Verification items for this drawing (mm, ordinates from the low corner). A direction names the side the tool comes from. Round coordinates to 2 decimals unless told otherwise and drop trailing zeros. Write each loop counter-clockwise with the first axis right and the second up, starting at its lowest first coordinate (ties: lowest second). Pieces come first, ordered by that corner, then holes.
Item 1: Cross-section at A-A (z = 27.5). Enter the section's corners in (x, y).
Item 2: Depth check by flat-ended pin: P1, Ø15, axis at x = 23.5, y = 23.5, coming from the -Z side; P2, Ø3.5, axis at x = 4.5, y = 26, coming from the +Z side; P3, Ø8, axis at y = 35.5, z = 17, coming from the -X side; P4, Ø4, axis at x = 44.5, z = 23, coming from the +Y side. Enter the tip coordinate at first touch or a pass-through.
Item 3: Cross-section at B-B (z = 37.5). State how many separate pieces and enclosed holes the cut face has, then the cut area to 3 significant figures.
Item 4: Cross-section at D-D (y = 10.5). Enter the section's corners in (x, z).
Item 5: Scan lines: probe 1 along Z at (x, y) = (20.5, 49.5); probe 2 along X at (y, z) = (26.5, 56.5); probe 3 along X at (y, z) = (47, 38) (1 decimal). Record each from-to range of solid material in increasing order.
Item 6: Draft check along Z on the marked faces 1, 2, 3 and 4. Enter one of: pulls with the +Z half, pulls with the -Z half, needs draft (parallel to the pull), parting line crosses it, or undercut.
Item 7: Access from +Z, -Z, +X, -X, +Y, -Y to the whole of each face (thin tool, end or side, straight path). Record for the marked faces 5 and 6.
Item 8: Cross-section at C-C (x = 35.5). Enter the section's corners in (y, z), then the cut area to 3 significant figures.
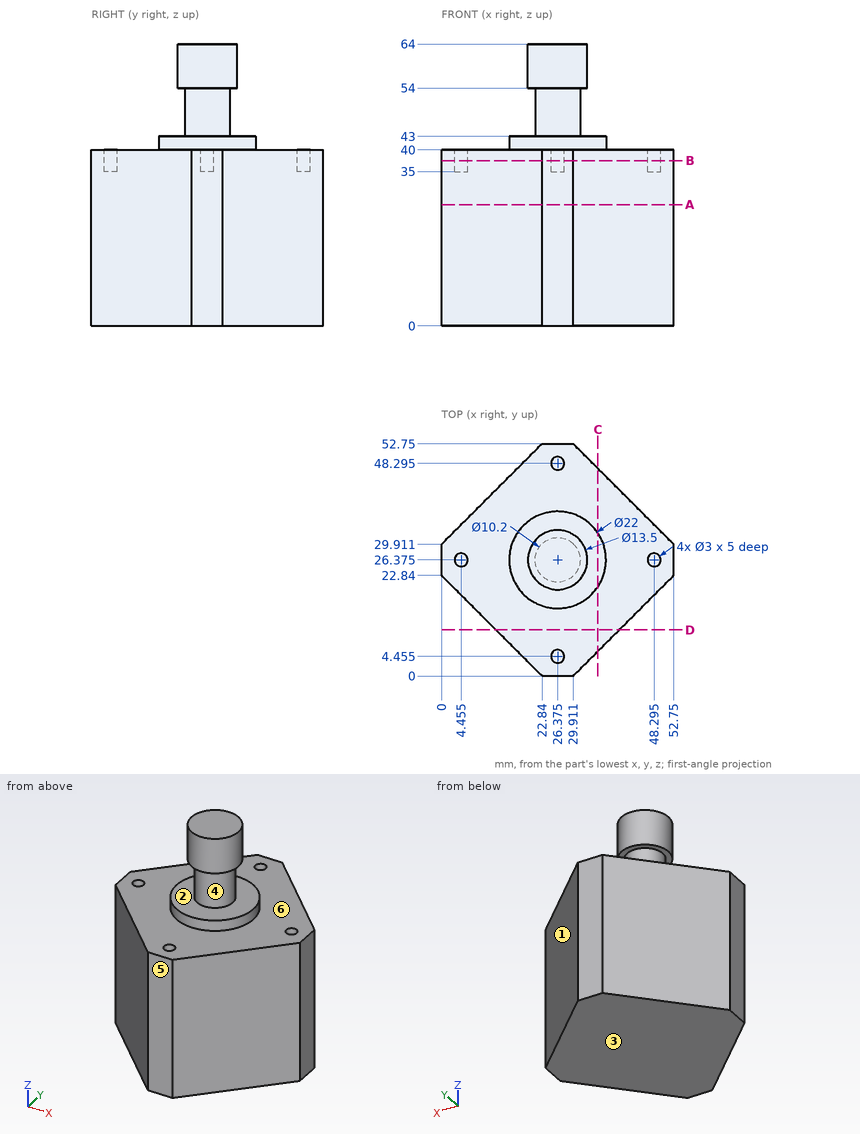
Resolved:
1. outline: (0, 22.84) - (22.84, 0) - (29.91, 0) - (52.75, 22.84) - (52.75, 29.91) - (29.91, 52.75) - (22.84, 52.75) - (0, 29.91) - close
2. P1: stops at z = 0
2. P2: stops at z = 40
2. P3: stops at x = 1.59
2. P4: stops at y = 40.16
3. separate pieces: 1
3. enclosed holes: 4
3. area: 1,710 mm2
4. outline: (12.34, 0) - (40.41, 0) - (40.41, 40) - (12.34, 40) - close
5. probe 1: z = 0 to 40
5. probe 2: x = 19.63 to 33.12
5. probe 3: x = 17.1 to 25.6, 27.1 to 35.7
6. face 1: needs draft
6. face 2: undercut
6. face 3: pulls with the -Z half
6. face 4: undercut
7. face 5: +Z, -Z, +X, -X, -Y
7. face 6: +Z
8. outline: (5.59, 0) - (47.16, 0) - (47.16, 40) - (32.52, 40) - (32.52, 43) - (20.23, 43) - (20.23, 40) - (5.59, 40) - close
8. area: 1,700 mm2
